Verification items for the finished model (mm, model axes). Face numbers are marked on the shaded views. A direction names the side the tool comes from. Round coordinates to 2 decimals unless told otherwise and drop trailing zeros. Order: outer loops, then holes, each group sorted by start corner. A loop starts at its lowest first (then second) coordinate and runs counter-clockwise, first axis right, second up. Notation, with made-up numbers: (-24, 10) -> (-10, 10) arc R29 ccw to (-10, 41) -> close; hole circle Ø7 at (82, -34). An arc over 180 degrees is marked (long way). Return JSON: item names as keys, results as strings. Group by question number.
Item 1: Depth check by flat-ended pin: pin 1 Ø8 at (y, z) = (50.5, -46) entering from -X; pin 2 Ø1 at (x, z) = (44.5, -24.5) entering from +Y; pin 3 Ø4 at (y, z) = (49, -69.5) entering from -X; pin 4 Ø1 at (x, z) = (-16.5, 31.5) entering from -Y. Enter the tip coordinate at first touch or a pass-through.
Item 2: Scan lines: probe 1 along Z at (x, y) = (-38, 39); probe 2 along X at (y, z) = (68, 25.5); probe 3 along Z at (x, y) = (-52, 47.5). Record each from-to range of solid material in increasing order. Write a range as from..to.
Item 3: Sectioned sample at D-D on z = -77.5. Record the cut outline in (x, y), plus the area to 3 significant figures.
Item 4: Sectioned sample at A-A on y = 40.5. Give the number of separate pieces and of enclosed holes in the cut face, plus the area to 3 significant figures.
Item 5: Sectioned sample at C-C on y = 83. Record the cut outline in (x, z).
Item 6: Draft check along X on the marked faces 1, 2 and 3. Enter one of: pulls with the +X half, pulls with the -X half, needs draft (parallel to the pull), parting line crosses it, or undercut.
Item 7: Access from +Z, -Z, +X, -X, +Y, -Y to the whole of each face (thin tool, end or side, straight path). Record for the marked faces 4 and 5.
Item 8: Sectioned sample at B-B on z = 71.5. Record the cut outline in (x, y).
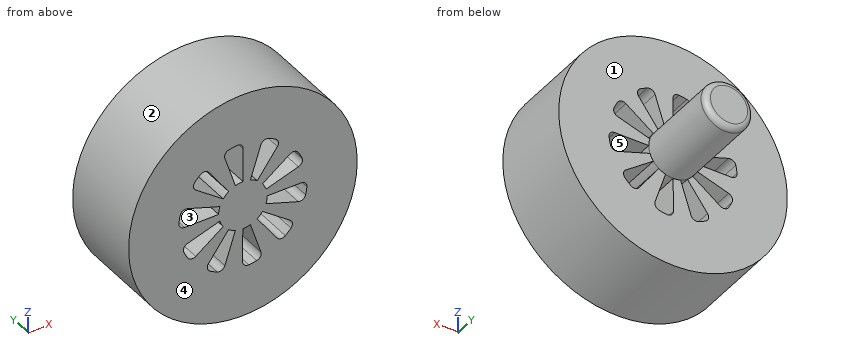
```python
from build123d import *

# Parameters (mm, degrees)
SKETCH1_R           = 101.6
BOSS_EXTRUDE1_DEPTH = 76.2
SKETCH2_R           = 21.59
BOSS_EXTRUDE2_DEPTH = 76.2
FILLET1_R           = 5.08


with BuildPart() as part:
    # Sketch1 → Boss-Extrude1 (new body)
    with BuildSketch(Plane(origin=(0, 0, 0), x_dir=(1, 0, 0), z_dir=(0, 1, 0))):
        Circle(SKETCH1_R)
        with BuildLine():
            Line((21.59, 0), (51.821602638, 0))
            ThreePointArc((51.821602638, 0), (55.584852402, 1.667617955), (56.877368749, 5.575609756))
            ThreePointArc((56.877368749, 5.575609756), (56.423832827, 9.081497074), (55.75440626, 12.552636482))
            ThreePointArc((55.75440626, 12.552636482), (53.300937227, 15.857706546), (49.204484901, 16.260294142))
            Line((49.204484901, 16.260294142), (20.499652171, 6.774390074))
            ThreePointArc((20.499652171, 6.774390074), (21.315670179, 3.430787784), (21.59, 0))
        make_face(mode=Mode.SUBTRACT)
        with BuildLine():
            Line((20.566453564, -6.568796527), (49.364825579, -15.766816277))
            ThreePointArc((49.364825579, -15.766816277), (52.442290076, -18.500350747), (52.484516777, -22.616321511))
            ThreePointArc((52.484516777, -22.616321511), (50.985809694, -25.818011346), (49.292019101, -28.920915493))
            ThreePointArc((49.292019101, -28.920915493), (45.949291463, -31.322825227), (41.92455721, -30.459973781))
            Line((41.92455721, -30.459973781), (17.466676909, -12.690283597))
            ThreePointArc((17.466676909, -12.690283597), (19.261305884, -9.753470953), (20.566453564, -6.568796527))
        make_face(mode=Mode.SUBTRACT)
        with BuildLine():
            Line((12.777568723, -17.402926119), (30.669480735, -41.771538773))
            ThreePointArc((30.669480735, -41.771538773), (31.552470563, -45.791902859), (29.167325768, -49.146613388))
            ThreePointArc((29.167325768, -49.146613388), (26.072940201, -50.855916954), (22.87879353, -52.37063401))
            ThreePointArc((22.87879353, -52.37063401), (18.762662945, -52.349013795), (16.013755891, -49.285272874))
            Line((16.013755891, -49.285272874), (6.671676909, -20.533310187))
            ThreePointArc((6.671676909, -20.533310187), (9.849777409, -19.212235294), (12.777568723, -17.402926119))
        make_face(mode=Mode.SUBTRACT)
        with BuildLine():
            Line((0.108086924, -21.589729438), (0.259436667, -51.82095322))
            ThreePointArc((0.259436667, -51.82095322), (-1.389320275, -55.592504489), (-5.290792323, -56.904569382))
            ThreePointArc((-5.290792323, -56.904569382), (-8.798906261, -56.468590815), (-12.273353548, -55.816550347))
            ThreePointArc((-12.273353548, -55.816550347), (-15.590665099, -53.379658372), (-16.013755891, -49.285272874))
            Line((-16.013755891, -49.285272874), (-6.671676909, -20.533310187))
            ThreePointArc((-6.671676909, -20.533310187), (-3.324031254, -21.332578752), (0.108086924, -21.589729438))
        make_face(mode=Mode.SUBTRACT)
        with BuildLine():
            Line((-12.602680406, -17.52998992), (-30.24970339, -42.076524866))
            ThreePointArc((-30.24970339, -42.076524866), (-33.800437989, -44.158658923), (-37.728007574, -42.926913988))
            ThreePointArc((-37.728007574, -42.926913988), (-40.309869596, -40.512182281), (-42.737496726, -37.942441587))
            ThreePointArc((-42.737496726, -37.942441587), (-43.988888982, -34.021087758), (-41.92455721, -30.459973781))
            Line((-41.92455721, -30.459973781), (-17.466676909, -12.690283597))
            ThreePointArc((-17.466676909, -12.690283597), (-15.228172958, -15.304602195), (-12.602680406, -17.52998992))
        make_face(mode=Mode.SUBTRACT)
        with BuildLine():
            Line((-20.499652171, -6.774390074), (-49.204484901, -16.260294142))
            ThreePointArc((-49.204484901, -16.260294142), (-53.300937227, -15.857706546), (-55.75440626, -12.552636482))
            ThreePointArc((-55.75440626, -12.552636482), (-56.423832827, -9.081497074), (-56.877368749, -5.575609756))
            ThreePointArc((-56.877368749, -5.575609756), (-55.584852402, -1.667617955), (-51.821602638, 0))
            Line((-51.821602638, 0), (-21.59, 0))
            ThreePointArc((-21.59, 0), (-21.315670179, -3.430787784), (-20.499652171, -6.774390074))
        make_face(mode=Mode.SUBTRACT)
        with BuildLine():
            Line((-20.566453564, 6.568796527), (-49.364825579, 15.766816277))
            ThreePointArc((-49.364825579, 15.766816277), (-52.442290076, 18.500350747), (-52.484516777, 22.616321511))
            ThreePointArc((-52.484516777, 22.616321511), (-50.985809694, 25.818011346), (-49.292019101, 28.920915493))
            ThreePointArc((-49.292019101, 28.920915493), (-45.949291463, 31.322825227), (-41.92455721, 30.459973781))
            Line((-41.92455721, 30.459973781), (-17.466676909, 12.690283597))
            ThreePointArc((-17.466676909, 12.690283597), (-19.261305884, 9.753470953), (-20.566453564, 6.568796527))
        make_face(mode=Mode.SUBTRACT)
        with BuildLine():
            Line((-12.777568723, 17.402926119), (-30.669480735, 41.771538773))
            ThreePointArc((-30.669480735, 41.771538773), (-31.552470563, 45.791902859), (-29.167325768, 49.146613388))
            ThreePointArc((-29.167325768, 49.146613388), (-26.072940201, 50.855916954), (-22.87879353, 52.37063401))
            ThreePointArc((-22.87879353, 52.37063401), (-18.762662945, 52.349013795), (-16.013755891, 49.285272874))
            Line((-16.013755891, 49.285272874), (-6.671676909, 20.533310187))
            ThreePointArc((-6.671676909, 20.533310187), (-9.849777409, 19.212235294), (-12.777568723, 17.402926119))
        make_face(mode=Mode.SUBTRACT)
        with BuildLine():
            Line((-0.108086924, 21.589729438), (-0.259436667, 51.82095322))
            ThreePointArc((-0.259436667, 51.82095322), (1.389320275, 55.592504489), (5.290792323, 56.904569382))
            ThreePointArc((5.290792323, 56.904569382), (8.798906261, 56.468590815), (12.273353548, 55.816550347))
            ThreePointArc((12.273353548, 55.816550347), (15.590665099, 53.379658372), (16.013755891, 49.285272874))
            Line((16.013755891, 49.285272874), (6.671676909, 20.533310187))
            ThreePointArc((6.671676909, 20.533310187), (3.324031254, 21.332578752), (-0.108086924, 21.589729438))
        make_face(mode=Mode.SUBTRACT)
        with BuildLine():
            Line((12.602680406, 17.52998992), (30.24970339, 42.076524866))
            ThreePointArc((30.24970339, 42.076524866), (33.800437989, 44.158658923), (37.728007574, 42.926913988))
            ThreePointArc((37.728007574, 42.926913988), (40.309869596, 40.512182281), (42.737496726, 37.942441587))
            ThreePointArc((42.737496726, 37.942441587), (43.988888982, 34.021087758), (41.92455721, 30.459973781))
            Line((41.92455721, 30.459973781), (17.466676909, 12.690283597))
            ThreePointArc((17.466676909, 12.690283597), (15.228172958, 15.304602195), (12.602680406, 17.52998992))
        make_face(mode=Mode.SUBTRACT)
    extrude(amount=BOSS_EXTRUDE1_DEPTH)

    # Sketch2 → Boss-Extrude2 (add)
    with BuildSketch(Plane(origin=(0, 76.2, 0), x_dir=(1, 0, 0), z_dir=(0, 1, 0))):
        Circle(SKETCH2_R)
    extrude(amount=BOSS_EXTRUDE2_DEPTH)

    # Fillet1
    fillet1_edges = [part.edges().sort_by_distance(p)[0] for p in [
        (-21.59, 152.4, 0),
    ]]
    fillet(fillet1_edges, radius=FILLET1_R)


solid = part.part
```
Recorded:
{
 "1": {"pin 1": "x = -92.51", "pin 2": "y = 76.2", "pin 3": "x = -75.94", "pin 4": "y = 0"},
 "2": {"probe 1": "-94.23..-27.61, -12.14..0, 12.56..27.61, 42.69..94.23", "probe 2": "-98.35..-35.1, -18.33..-8.29, 0.13..8.29, 18.72..35.1, 51.15..98.35", "probe 3": "-87.28..-23.71, -17.72..0, 16.37..87.28"},
 "3": {"outline": "(-65.7, 0) -> (65.7, 0) -> (65.7, 76.2) -> (-65.7, 76.2) -> close", "area": "10,000 mm²"},
 "4": {"separate pieces": "1", "enclosed holes": "10", "area": "28,100 mm²"},
 "5": {"outline": "circle Ø43.18 at (0, 0)"},
 "6": {"face 1": "needs draft", "face 2": "parting line crosses it", "face 3": "undercut"},
 "7": {"face 4": "+Z, -Z, +X, -X, -Y", "face 5": "+Y, -Y"},
 "8": {"outline": "(-72.18, 0) -> (72.18, 0) -> (72.18, 76.2) -> (-72.18, 76.2) -> close"}
}
